Source: CAD feature listing. Evaluate the final solid. Frame: model axes, mm. A direction names the side the tool comes from. Give positions to 0.01 mm unless a question says otherwise; leave off trailing zeros. Write each loop counter-clockwise with the first axis right and the second up, starting at its lowest first coordinate (ties: lowest second). Pieces come first, ordered by that corner, then holes. Notation, with made-up numbers: (41.25, -39) -> (77.25, -39) arc R14 ccw to (77.25, -21) -> close; hole circle Ø6 at (80.5, 21). An arc over 180 degrees is marked (long way). Use a Markdown table: item, result. Add a question column.
```python
from build123d import *

# Parameters (mm, degrees)
SKETCH2_W = 0.37
SKETCH2_H = 1
SKETCH3_W = 0.4
SKETCH3_H = 6
SKETCH4_W = 3.1
SKETCH4_H = 4.5


with BuildPart() as part:
    # Sketch1 → Body (revolve)
    with BuildSketch(Plane(origin=(0, 0, 0), x_dir=(-1, 0, 0), z_dir=(0, 1, 0)), mode=Mode.PRIVATE) as body_sk:
        Polygon((0, 30.34), (-0.74, 30.01), (-2.67, 27.87), (-3.08, 26.8), (-2.51, 25.58), (-1.98, 24.43), (-2.7, 23.15), (-3.08, 22.47), (-3.15, 21.84), (-3.15, 0), (-4.48, 0), (-4.48, -0.6), (-5.6, -0.6), (-6.35, -1.35), (-6.35, -38), (-4.8, -44.5), (-4.8, -46), (0, -46), align=None)
    revolve(body_sk.sketch.rotate(Axis((0, 0, -200), (0, 0, 1)), 180), axis=Axis((0, 0, -200), (0, 0, 1)))

    # Sketch2 → Insulators (revolve, cut)
    with BuildSketch(Plane(origin=(0, 0, 0), x_dir=(-1, 0, 0), z_dir=(0, 1, 0)), mode=Mode.PRIVATE) as insulators_sk:
        with Locations((-3.215, 21.8)):
            Rectangle(SKETCH2_W, SKETCH2_H)
        with Locations((-3.215, 15.3)):
            Rectangle(SKETCH2_W, SKETCH2_H)
    revolve(insulators_sk.sketch.rotate(Axis((0, 0, -200), (0, 0, 1)), 180), axis=Axis((0, 0, -200), (0, 0, 1)), mode=Mode.SUBTRACT)

    # Sketch3 → Grip (revolve, cut)
    with BuildSketch(Plane(origin=(0, 0, 0), x_dir=(-1, 0, 0), z_dir=(0, 1, 0)), mode=Mode.PRIVATE) as grip_sk:
        with Locations((-6.4, -13)):
            Rectangle(SKETCH3_W, SKETCH3_H)
        with Locations((-6.4, -35)):
            Rectangle(SKETCH3_W, SKETCH3_H)
    revolve(grip_sk.sketch.rotate(Axis((0, 0, -200), (0, 0, 1)), 180), axis=Axis((0, 0, -200), (0, 0, 1)), mode=Mode.SUBTRACT)

    # Sketch4 → CableBore (revolve, cut)
    with BuildSketch(Plane(origin=(0, 0, 0), x_dir=(-1, 0, 0), z_dir=(0, 1, 0))):
        with Locations((-1.55, -44.25)):
            Rectangle(SKETCH4_W, SKETCH4_H)
    revolve(axis=Axis((0, 0, -200), (0, 0, 1)), mode=Mode.SUBTRACT)


solid = part.part
```
(1) Cut plane A-A on z = 3. Return the cut outline in (x, y).
(2) Material intervals for L1, parallel to Y at x = 0, z = -43.5; L2, parallel to X at y = -3, z = -18.5; L3, parallel to Z at x = 0.5, y = -0.5, sorted ascending.
(3) Access query for faces 1 (the cylindrical face through (3.555, 2.726, -0.304)), 2 (the cylindrical face through (-5.9, -1.9, -13)), 3 (the cylindrical face through (-2.93, 5.634, -24.112)). Directions: +Z, -Z, +X, -X, +Y, -Y. A direction counts if a zero-diameter tool reaches every point of the face in a straight line with its end or side. Return the directions, or none.
(4) Mould query, pull axis Z, two halves, no side actions, for faces 4 (the cylindrical face through (0.683, 3.075, 18.512)), 5 (the conical face through (4.14, 3.18, -42.74)), 6 (the cylindrical face through (0.657, 2.958, 15.307)). Classes: +Z half, -Z half, draft (parallel to the pull), parting line (faces both ways), or undercut.
(5) First-contact query: pin 1 Ø4 at (y, z) = (3, -19) entering from +X; pin 2 Ø1.5 at (y, z) = (3.5, 5.5) entering from +X; pin 3 Ø1.9 at (x, y) = (1, 1.5) entering from +Z. Flat tips, straight axial feed; report the tip coordinate or a pass-through.
Output:
| question | item | result |
|---|---|---|
| 1 | outline | circle Ø6.3 at (0, 0) |
| 2 | L1 | -5.04 to -3.1, 3.1 to 5.04 |
| 2 | L2 | -5.6 to 5.6 |
| 2 | L3 | -42 to 30.02 |
| 3 | face 1 | +Z |
| 3 | face 2 | none |
| 3 | face 3 | +Z, -Z |
| 4 | face 4 | draft |
| 4 | face 5 | -Z half |
| 4 | face 6 | undercut |
| 5 | pin 1 | x = 6.27 |
| 5 | pin 2 | x = 1.54 |
| 5 | pin 3 | z = 29.88 |
